Could you check a few things on this model? Use its own coordinates, in mm. Face numbers are marked on the shaded views. A direction names the side the tool comes from. Round coordinates to 2 decimals unless told otherwise and drop trailing zeros. Order: outer loops, then holes, each group sorted by start corner. A loop starts at its lowest first (then second) coordinate and runs counter-clockwise, first axis right, second up. Notation, with made-up numbers: M 71,79.5 L 104,79.5 A24 cw 104,101.5 Z; hole C -10.5,-26.5 d9. An arc over 180 degrees is marked long. Write each question's results on one line, items separated by ' | '. Start each with the question number.
1. Suppose I cut it at D-D on x = 28.5. Write out the boundary of the cut face in (y, z), and give its area (3 significant figures).
2. Suppose I cut it at C-C on x = 4. Write out the boundary of the cut face in (y, z).
3. Suppose I cut it at B-B on z = -42. Write out the boundary of the cut face in (x, y).
4. We'd pull the mould along Z, two halves only. Please class the marked faces 3, 4, 5 and 6: released by +Z, released by -Z, zero draft, split by the parting line, or undercut.
5. For the marked faces 1 and 2, which set-ups out of +Z, -Z, +X, -X, +Y, -Y let a thin tool reach every point of the face, with its end or its side?
6. Suppose I cut it at A-A on y = 9. Write out the boundary of the cut face in (x, z), and give its area (3 significant figures).
7. Please list where these lines run through material, in increasing order: L1, parallel to X at y = 0.75, z = -42; L2, parallel to Z at x = 1, y = 1.5; L3, parallel to Y at x = 39, z = -27.
8. I'm going to push a flat-ended pin straight in: pin 1 (3 mm diameter, centred on x = 37.5, z = -33.5, fed in from +Y). Where does the tip first touch, or does it pass through?
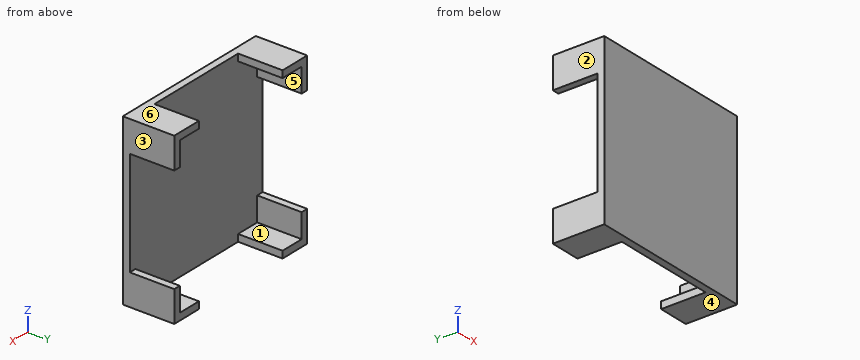
Autodesk Inventor part; units mm, degrees
ref_plane "YZ Plane" through (0, 0, 0) normal (1, 0, 0) x (0, 1, 0)
ref_plane "XZ Plane" through (0, 0, 0) normal (0, 1, 0) x (-1, 0, 0)
ref_plane "XY Plane" through (0, 0, 0) normal (0, 0, 1) x (1, 0, 0)
sketch "Sketch1" plane through (0, 0, 0) normal (0, 1, 0) x (-1, 0, 0)
  line L0 (0, 0) -> (-44, 0)
  line L1 (-44, 0) -> (-44, -44)
  line L2 (-44, -44) -> (0, -44)
  line L3 (0, -44) -> (0, 0)
  line L4 (2, 2) -> (-46, 2)
  line L5 (-46, 2) -> (-46, -46)
  line L6 (-46, -46) -> (2, -46)
  line L7 (2, -46) -> (2, 2)
  dimension "d0" = 44
  dimension "d1" = 44
  dimension "d2" = 48
  dimension "d3" = 48
  dimension "d4" = 2
  dimension "d5" = 2
extrude "Extrusion1" add sketch "Sketch1" along normal blind 12.7
sketch "Sketch2" plane through (0, 0, 0) normal (0, -1, 0) x (1, 0, 0)
  line L0 (46, 2) -> (46, -46)
  line L1 (-2, 2) -> (46, 2)
  line L2 (-2, -46) -> (-2, 2)
  line L3 (46, -46) -> (-2, -46)
  point P0 (0, 0)
extrude "Extrusion2" add sketch "Sketch2" along normal blind 2
sketch "Sketch3" plane through (0, 0, 0) normal (0, 1, 0) x (1, 0, 0)
  line L0 (-2, -2) -> (46, -2)
  line L1 (-2, 46) -> (-2, -2)
  line L2 (46, 46) -> (-2, 46)
  line L3 (46, -2) -> (46, 46)
  line L4 (37.11, -2) -> (6.89, -2)
  line L5 (6.89, -2) -> (6.89, 46)
  line L6 (6.89, 46) -> (37.11, 46)
  line L7 (37.11, 46) -> (37.11, -2)
  line L8 (-2, -2) -> (-2, 46)
  line L9 (-2, 6.89) -> (46, 6.89)
  line L10 (46, 6.89) -> (46, 37.11)
  line L11 (46, 37.11) -> (-2, 37.11)
  line L12 (-2, 37.11) -> (-2, 6.89)
  point P0 (0, 0)
  point P1 (37.11, 37.11)
  point P2 (37.11, 6.89)
  point P3 (6.89, 6.89)
  point P4 (6.89, 37.11)
  point P5 (-2, 37.11)
  dimension "d10" = 8.89
  dimension "d11" = 8.89
  dimension "d12" = 8.89
  dimension "d13" = 8.89
extrude "Extrusion3" cut sketch "Sketch3" along normal blind 2 contours L5 L9 L7 L0 | L1 L11 L5 L9 | L7 L11 L3 L9 | L5 L2 L7 L11
extrude "Extrusion4" cut sketch "Sketch3" along normal blind 76.2 contours L5 L9 L7 L0 | L1 L11 L5 L9 | L7 L11 L3 L9 | L5 L2 L7 L11
properties part number "servoBracket"
Filled sheet:
1) outline: M -2,-46 L 0,-46 L 0,2 L -2,2 Z | area: 96.0 mm^2
2) outline: M -2,-46 L 12.7,-46 L 12.7,-44 L 0,-44 L 0,0 L 12.7,0 L 12.7,2 L -2,2 Z
3) outline: M -2,-2 L 46,-2 L 46,12.7 L 44,12.7 L 44,0 L 0,0 L 0,12.7 L -2,12.7 Z
4) face 3: zero draft | face 4: released by -Z | face 5: undercut | face 6: released by +Z
5) face 1: +Y | face 2: +Z, -Z, -X, +Y, -Y
6) outline: M -2,-46 L 6.89,-46 L 6.89,-44 L 0,-44 L 0,-37.11 L -2,-37.11 Z; M -2,-6.89 L 0,-6.89 L 0,0 L 6.89,0 L 6.89,2 L -2,2 Z; M 37.11,-46 L 46,-46 L 46,-37.11 L 44,-37.11 L 44,-44 L 37.11,-44 Z; M 37.11,0 L 44,0 L 44,-6.89 L 46,-6.89 L 46,2 L 37.11,2 Z | area: 126 mm^2
7) L1: x = -2 to 0, 44 to 46 | L2: z = -46 to -44, 0 to 2 | L3: y = -2 to 0
8) pin 1: stops at y = 0
